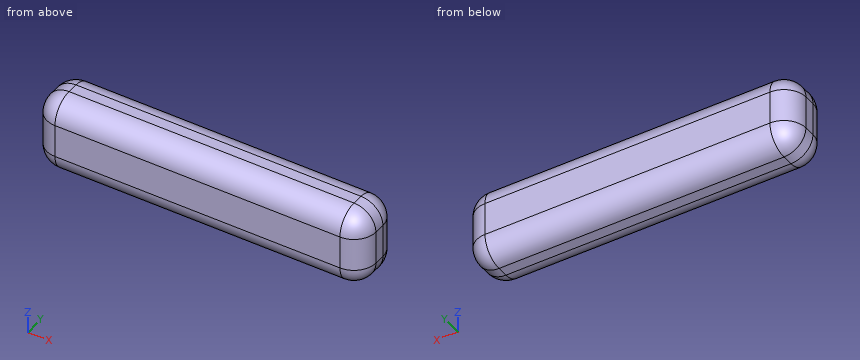
from build123d import *

# Parameters (mm, degrees)
F0_W     = 76.2
F0_H     = 12.7
F1_DEPTH = 17.78
F2_R     = 5.08
F3_R     = 5.08
F4_R     = 5.08


with BuildPart() as f1:
    # F0 (on Top) → F1 (new body)
    with BuildSketch(Plane.XY):
        Rectangle(F0_W, F0_H)
    extrude(amount=F1_DEPTH)

    # F2
    f2_edges = [f1.edges().sort_by_distance(p)[0] for p in [
        (0, 6.35, 17.78),
        (0, -6.35, 17.78),
        (0, 6.35, 0),
        (0, -6.35, 0),
    ]]
    fillet(f2_edges, radius=F2_R)

    # F3
    f3_edges = [f1.edges().sort_by_distance(p)[0] for p in [
        (-38.1, 0, 17.78),
        (-38.1, -4.862102, 16.292102),
        (-38.1, 4.862102, 16.292102),
        (-38.1, 6.35, 8.89),
        (-38.1, -6.35, 8.89),
        (-38.1, -4.862102, 1.487898),
        (-38.1, 0, 0),
        (-38.1, 4.862102, 1.487898),
    ]]
    fillet(f3_edges, radius=F3_R)

    # F4
    f4_edges = [f1.edges().sort_by_distance(p)[0] for p in [
        (38.1, -4.862102, 16.292102),
        (38.1, 0, 17.78),
        (38.1, 4.862102, 16.292102),
        (38.1, 6.35, 8.89),
        (38.1, 4.862102, 1.487898),
        (38.1, 0, 0),
        (38.1, -4.862102, 1.487898),
        (38.1, -6.35, 8.89),
    ]]
    fillet(f4_edges, radius=F4_R)


solid = f1.part
Input: part model. Units: mm. Frame: model coordinates. Give positions to 0.01 mm unless a question says otherwise; leave off trailing zeros. Write each loop counter-clockwise with the first axis right and the second up, starting at its lowest first coordinate (ties: lowest second). Pieces come first, ordered by that corner, then holes. Notation, with made-up numbers: M 58.25,-12.75 L 86.25,-12.75 A16 cw 86.25,-3.75 Z; hole C 57,34.5 d7. An arc over 180 degrees is marked long. Write item = value, one per line. Start each with the question number.
1) Cut plane B-B on z = 7.75. Return the cut outline in (x, y).
2) Cut plane A-A on x = -24.5. Return the cut outline in (y, z), then the cut area to 3 significant figures.
3) Material intervals for line 1 along Z through (x, y) = (-21, 1.5); line 2 along Y through (x, z) = (-3.5, 13); line 3 along X through (y, z) = (-1.5, 12.75), sorted ascending. Write a range as [from, to].
4) First-contact query: pin 1 Ø1.5 at (y, z) = (4.5, 8) entering from +X; pin 2 Ø1.5 at (x, y) = (4.5, -2.5) entering from +Z; pin 3 Ø1.5 at (x, y) = (-10, 4.5) entering from -Z. Flat tips, straight axial feed; report the tip coordinate or a pass-through.
Solved:
q1.outline = M -38.1,-1.27 A5.08 ccw -33.02,-6.35 L 33.02,-6.35 A5.08 ccw 38.1,-1.27 L 38.1,1.27 A5.08 ccw 33.02,6.35 L -33.02,6.35 A5.08 ccw -38.1,1.27 Z
q2.outline = M -6.35,5.08 A5.08 ccw -1.27,0 L 1.27,0 A5.08 ccw 6.35,5.08 L 6.35,12.7 A5.08 ccw 1.27,17.78 L -1.27,17.78 A5.08 ccw -6.35,12.7 Z
q2.area = 204 mm2
q3.line_1 = [0.01, 17.77]
q3.line_2 = [-6.34, 6.34]
q3.line_3 = [-38.09, 38.09]
q4.pin_1 = 37.45
q4.pin_2 = 17.76
q4.pin_3 = 0.65
